```python
from build123d import *

# Parameters (mm, degrees)
SKETCH2_R           = 4
BOSS_EXTRUDE1_DEPTH = 4


with BuildPart() as part:
    # Sketch2 → Boss-Extrude1 (new body)
    with BuildSketch(Plane.XY):
        with BuildLine():
            Line((-48.202812442, -6.461632916), (-48.202812442, -13.961632916))
            Line((-48.202812442, -13.961632916), (91.797187558, -13.961632916))
            ThreePointArc((91.797187558, -13.961632916), (104.297187558, -1.461632916), (91.797187558, 11.038367084))
            Line((91.797187558, 11.038367084), (-48.202812442, 11.038367084))
            Line((-48.202812442, 11.038367084), (-48.202812442, 3.538367084))
            Line((-48.202812442, 3.538367084), (-52.202812442, 3.538367084))
            Line((-52.202812442, 3.538367084), (-52.202812442, -6.461632916))
            Line((-52.202812442, -6.461632916), (-48.202812442, -6.461632916))
        make_face()
        with Locations((91.797187558, -1.461632916)):
            Circle(SKETCH2_R, mode=Mode.SUBTRACT)
    extrude(amount=BOSS_EXTRUDE1_DEPTH)


solid = part.part
```
Model file for the job. Use its own axes, mm. A direction names the side the tool comes from. Give positions to 0.01 mm unless a question says otherwise; leave off trailing zeros. Write each loop counter-clockwise with the first axis right and the second up, starting at its lowest first coordinate (ties: lowest second). Pieces come first, ordered by that corner, then holes. Notation, with made-up numbers: (-6, -22) - (29, -22) arc R29 ccw to (29, 6) - close; hole circle Ø7 at (42, 28.5). An arc over 180 degrees is marked (long way). One line per question, with ' | ' between items. Start each with the question number.
(1) Slice it at D-D on y = -12. Write the cut outline in (x, z), plus the area to 3 significant figures.
(2) 3-axis set-ups, long thin cutter, end or side, ignore diameter. For faces 5 (the face through (-50, 3.538, 2)), 6 (the face through (25, -1, 0)), 7 (the face through (-50, -6.462, 2)): which of +Z, -Z, +X, -X, +Y, -Y reach the whole face in a straight line?
(3) Wall check: line 1 along X through (y, z) = (-1, 0.7); line 2 along X through (y, z) = (1.5, 1.45); line 3 along X through (y, z) = (8.5, 3.5). Give the ranges that are in metal, low to high. Write a range as from..to.
(4) Slice it at B-B on z = 1.3. Write the cut outline in (x, y), plus the area to 3 significant figures.
(5) Pin check, flat tips, straight feed: P1, Ø1, axis at y = 1.5, z = 3, coming from the +X side; P2, Ø1.5, axis at y = -0.5, z = 3, coming from the +X side; P3, Ø2, axis at x = -49.5, z = 1.5, coming from the -Y side. Stop position of each tip, or through.
(6) Slice it at A-A on y = -3.5. Write the cut outline in (x, z).
(7) Slice it at C-C on y = 7.25. Write the cut outline in (x, z).
(8) Two-plate mould, pull along X, no slides. Class faces 1 (the face through (87.8, -1.3, 2)), 2 (the face through (25, -1, 4)), 3 (the face through (104.294, -1.737, 1.972)), 4 (the face through (-52.203, -1, 2)): +X half, -X half, draft (parallel to the pull), parting line (faces both ways), or undercut.
Results below:
1) outline: (-48.2, 0) - (98.52, 0) - (98.52, 4) - (-48.2, 4) - close | area: 587 mm^2
2) face 5: +Z, -Z, -X, +Y | face 6: -Z, +X, -X, +Y, -Y | face 7: +Z, -Z, -X, -Y
3) line 1: -52.2..87.82, 95.77..104.29 | line 2: -52.2..89.11, 94.49..103.94 | line 3: -48.2..99.35
4) outline: (-52.2, -6.46) - (-48.2, -6.46) - (-48.2, -13.96) - (91.8, -13.96) arc R12.5 ccw to (91.8, 11.04) - (-48.2, 11.04) - (-48.2, 3.54) - (-52.2, 3.54) - close; hole circle Ø8 at (91.8, -1.46) | area: 3,740 mm^2
5) P1: x = 104.05 | P2: x = 104.3 | P3: y = -6.46
6) outline: (-52.2, 0) - (88.36, 0) - (88.36, 4) - (-52.2, 4) - close; (95.24, 0) - (104.13, 0) - (104.13, 4) - (95.24, 4) - close
7) outline: (-48.2, 0) - (100.76, 0) - (100.76, 4) - (-48.2, 4) - close
8) face 1: undercut | face 2: draft | face 3: +X half | face 4: -X half
